The figure shows three views and two pictorial views of one solid part (mm, origin at its lowest corner). Answer the questions. Round coordinates to 2 decimals unless told otherwise and drop trailing zeros. Order: outer loops, then holes, each group sorted by start corner. A loop starts at its lowest first (then second) coordinate and runs counter-clockwise, first axis right, second up. Notation, with made-up numbers: (-18, 78) - (-13, 78) arc R14 ccw to (-13, 87) - close; hole circle Ø4 at (25, 49.5). An arc over 180 degrees is marked (long way). Use CSV: the item, a comma, the result in double quotes.
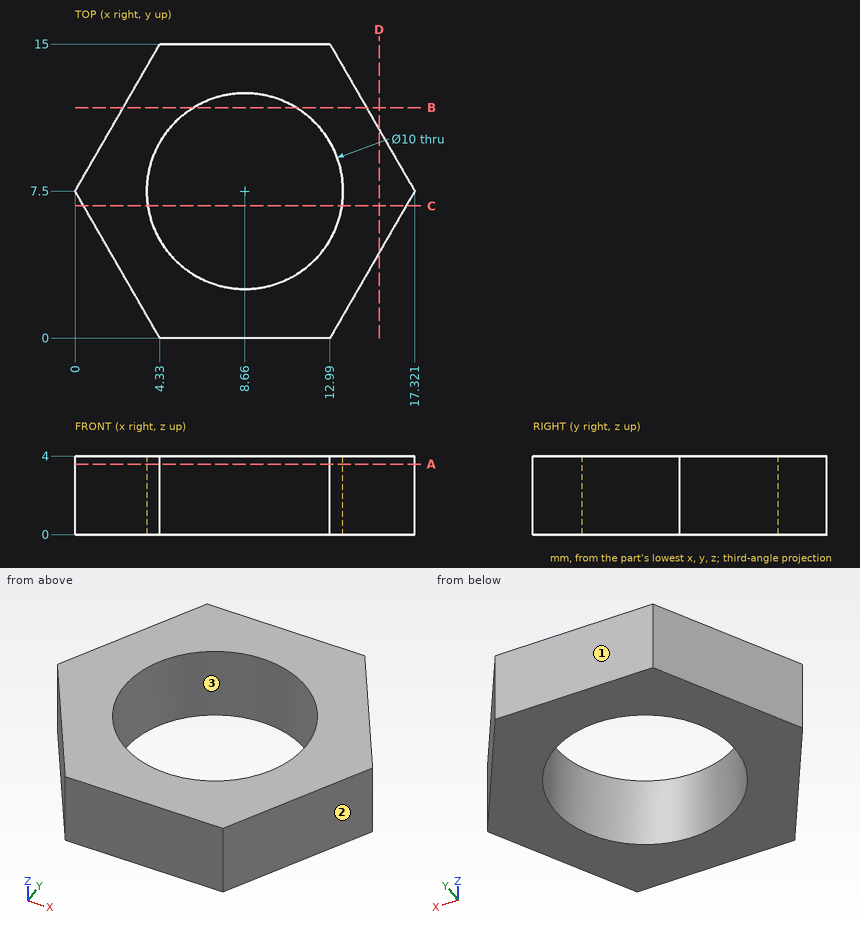
(1) Find the intervals of material crossed by L1, parallel to Y at x = 8.5, z = 1; L2, parallel to X at y = 11, z = 0.65; L3, parallel to X at y = 6, z = 1.25 (1 decimal), in increasing order. Write a range as from..to.
Findings below:
L1,"y = 0..2.5, 12.5..15"
L2,"x = 2.02..5.09, 12.23..15.3"
L3,"x = 0.9..3.9, 13.4..16.5"
(2) Find section B-B (y = 11.75). Determine the outline of the cut face in (x, z) (1 decimal), and give its area (3 significant figures).
Findings below:
outline,"(2.5, 0) - (6, 0) - (6, 4) - (2.5, 4) - close; (11.3, 0) - (14.9, 0) - (14.9, 4) - (11.3, 4) - close"
area,"28.6 mm²"
(3) Find section A-A (z = 3.6). Determine the outline of the cut face in (x, y), and give its area (3 significant figures).
Findings below:
outline,"(0, 7.5) - (4.33, 0) - (12.99, 0) - (17.32, 7.5) - (12.99, 15) - (4.33, 15) - close; hole circle Ø10 at (8.66, 7.5)"
area,"116 mm²"
(4) Find section D-D (x = 15.5). Determine the outline of the cut face in (y, z).
Findings below:
outline,"(4.35, 0) - (10.65, 0) - (10.65, 4) - (4.35, 4) - close"
(5) The mould has two halves that part along X. Classify the marked faces 1, 2 and 3: released by +X, released by -X, zero draft, split by the parting line, or undercut.
Findings below:
face 1,"zero draft"
face 2,"released by +X"
face 3,"undercut"
(6) Each of these flat-tipped pins is pushed along its axis until it touches: pin 1 (6 mm diameter, centred on x = 11.5, y = 12, fed in from -Z); pin 2 (1 mm diameter, centred on y = 5.5, z = 2, fed in from -X) (1 decimal); pin 3 (1.5 mm diameter, centred on y = 10, z = 0.5, fed in from -X). Where does it stop, or does it pass through?
Findings below:
pin 1,"stops at z = 0"
pin 2,"stops at x = 0.9"
pin 3,"stops at x = 1.01"
(7) Find section C-C (y = 6.75). Determine the outline of the cut face in (x, z).
Findings below:
outline,"(0.43, 0) - (3.72, 0) - (3.72, 4) - (0.43, 4) - close; (13.6, 0) - (16.89, 0) - (16.89, 4) - (13.6, 4) - close"
